from build123d import *

# Parameters (mm, degrees)
F1_DEPTH  = 25.4
F2_W      = 35.56
F2_H      = 27.2373445332
F3_DEPTH  = 11.7755213211
F5_DEPTH  = 10.16
F6_W      = 50.8
F6_H      = 36.2164959553
F7_DEPTH  = 21.4742356462
F8_R      = 12.7
F9_W      = 10.16
F9_H      = 3.048
F10_DEPTH = 0.508
F11_R     = 0.9525
F12_DEPTH = 38.101
F13_R     = 0.9525
F14_DEPTH = 38.101


with BuildPart() as f1:
    # F0 (on Right) → F1 (new body, symmetric)
    with BuildSketch(Plane.YZ):
        with BuildLine():
            Line((18.8676062971, 11.7745213211), (0, 0))
            Line((0, 0), (-35.1084388614, -8.89))
            Line((-35.1084388614, -8.89), (-40.9786602931, -16.51))
            Line((-40.9786602931, -16.51), (-32.1733296278, -16.51))
            ThreePointArc((-32.1733296278, -16.51), (-22.0133296278, -6.35), (-11.8533296278, -16.51))
            Line((-11.8533296278, -16.51), (44.4567567372, -16.51))
            ThreePointArc((44.4567567372, -16.51), (54.6167567372, -6.35), (64.7767567372, -16.51))
            Line((64.7767567372, -16.51), (74.9908098316, -11.6867008752))
            Line((74.9908098316, -11.6867008752), (74.9908098316, 0))
            Line((74.9908098316, 0), (64.5470768213, 0))
            Line((64.5470768213, 0), (37.3096317053, 11.7745213211))
            Line((37.3096317053, 11.7745213211), (18.8676062971, 11.7745213211))
        make_face()
    extrude(amount=F1_DEPTH, both=True)

    # F2 (on face) → F3 (cut, through all)
    with BuildSketch(Plane.XY):
        with Locations((0, 50.9284045547)):
            Rectangle(F2_W, F2_H)
    extrude(amount=F3_DEPTH, mode=Mode.SUBTRACT)

    # F4 (on face) → F5 (join)
    with BuildSketch(Plane(origin=(0, 0, -16.51), x_dir=(1, 0, 0), z_dir=(0, 0, -1))):
        Polygon((-12.7, -72.8133333333), (0, -72.8133333333), (12.7, -72.8133333333), (12.7, 32.1743115783), (-12.7, 32.1743115783), align=None)
    extrude(amount=-F5_DEPTH)

    # F6 (on face) → F7 (cut, through all)
    with BuildSketch(Plane(origin=(0, 0, 0), x_dir=(1, 0, 0), z_dir=(0, -0.2454682532, 0.96940463))):
        with Locations((0, -18.1082479777)):
            Rectangle(F6_W, F6_H)
    extrude(amount=F7_DEPTH, mode=Mode.SUBTRACT)

    # F8
    f8_edges = [f1.edges().sort_by_distance(p)[0] for p in [
        (0, -35.108439, -8.89),
    ]]
    fillet(f8_edges, radius=F8_R)

    # F9 (on face) → F10 (cut)
    with BuildSketch(Plane(origin=(0, 74.9908098316, 0), x_dir=(-1, 0, 0), z_dir=(0, 1, 0))):
        with Locations((0, -4.6856853668)):
            Rectangle(F9_W, F9_H)
    extrude(amount=-F10_DEPTH, mode=Mode.SUBTRACT)

    # F11 (on face) → F12 (cut, through all)
    with BuildSketch(Plane.YZ.offset(12.7)):
        with Locations((-22.0133296278, -15.24)):
            Circle(F11_R)
    extrude(amount=-F12_DEPTH, mode=Mode.SUBTRACT)

    # F13 (on face) → F14 (cut, through all)
    with BuildSketch(Plane.YZ.offset(12.7)):
        with Locations((54.6167567372, -15.24)):
            Circle(F13_R)
    extrude(amount=-F14_DEPTH, mode=Mode.SUBTRACT)


solid = f1.part
Build history of the part. All positions in model axes, mm. A direction names the side the tool comes from. Coordinates: 2 decimals unless noted, no trailing zeros. Order: outer loops, then holes, each group sorted by start corner. A loop starts at its lowest first (then second) coordinate and runs counter-clockwise, first axis right, second up. Notation, with made-up numbers: (17, -11) - (41, -11) arc R24 cw to (41, 5) - close; hole circle Ø1 at (55, 81). An arc over 180 degrees is marked (long way). Put each result on its own line as item: value.
1. Saw through at B-B (y = 47.5). Write the cut outline in (x, z), and give its area (3 significant figures).
Answer sheet:
outline: (-25.4, -9.26) - (-12.7, -9.26) - (-12.7, -16.51) - (12.7, -16.51) - (12.7, -9.26) - (25.4, -9.26) - (25.4, 7.37) - (17.78, 7.37) - (17.78, 0) - (-17.78, 0) - (-17.78, 7.37) - (-25.4, 7.37) - close
area: 767 mm^2
2. Tool access for faces 1 (the face through (0, 72.813, -15)), 2 (the face through (0, 28, 11.775)), 3 (the face through (-18.961, -22.237, -6.352)), 4 (the face through (19.139, 54.393, -6.352)), 5 (the face through (17.78, 48, 4)): list every direction of +Z, -Z, +X, -X, +Y, -Y with a clear straight run to the whole face (end or side of a thin tool).
Answer sheet:
face 1: -Z, +X, -X, +Y
face 2: +Z, +X, -X, +Y, -Y
face 3: -Z, -X
face 4: -Z, +X
face 5: +Z, +Y
3. Pull direction Z, two halves, no side cores. Call faces 6 (the face through (0, 74.483, -5)), 7 (the face through (-12.7, 71, -15)), 8 (the face through (19.139, -22.237, -6.352)): pulls with the +Z half, pulls with the -Z half, needs draft (parallel to the pull), parting line crosses it, or undercut.
Answer sheet:
face 6: undercut
face 7: needs draft
face 8: pulls with the -Z half
4. Drop flat-ended pins along their axis: P1, Ø4, axis at x = 2, z = -14.5, coming from the +Y side; P2, Ø3, axis at y = 59.5, z = -11, coming from the +X side; P3, Ø4, axis at x = -8, z = 2.5, coming from the +Y side; P4, Ø1.7, axis at y = -22.01, z = -15.24, coming from the +X side. Give the stop position or say it passes through.
Answer sheet:
P1: stops at y = 73.27
P2: stops at x = 12.7
P3: stops at y = 37.31
P4: passes through
5. Saw through at D-D (x = 7.5). Give the number of separate pieces and of enclosed holes in the cut face, and give its area (3 significant figures).
Answer sheet:
separate pieces: 1
enclosed holes: 2
area: 2,000 mm^2
6. Saw through at C-C (z = 7.25). Write the cut outline in (x, y), and give its area (3 significant figures).
Answer sheet:
outline: (-25.4, 11.62) - (25.4, 11.62) - (25.4, 47.78) - (17.78, 47.78) - (17.78, 37.31) - (-17.78, 37.31) - (-17.78, 47.78) - (-25.4, 47.78) - close
area: 1,460 mm^2
7. Probe line 1 along X through (y, z) = (46, 5); line 2 along Z through (x, y) = (-3, 42); line 3 along X through (y, z) = (54.5, -10.5). List the from-to ranges inside material, lowest first. Write a range as [from, to].
Answer sheet:
line 1: x = [-25.4, -17.78], [17.78, 25.4]
line 2: z = [-16.51, 0]
line 3: x = [-12.7, 12.7]
